```python
from build123d import *

# Parameters (mm, degrees)
SKETCH_1_W             = 26
SKETCH_1_H             = 82
EXTRUDE_1_DEPTH        = 9
CHAMFER_1_SIZE         = 5
CUT_EXTRUDE_1_DEPTH    = 87.492774265
SKETCH_3_OUTSIDE_W     = 45.298
SKETCH_3_OUTSIDE_H     = 101.298
SKETCH_3_OUTSIDE_W_2   = 20
SKETCH_3_OUTSIDE_H_2   = 55
CUT_EXTRUDE_2_DEPTH    = 3
SKETCH_4_W             = 12.420254628
SKETCH_4_H             = 10
CUT_EXTRUDE_3_DEPTH    = 87.492774265
PATTERN_LINEAR_1_COUNT = 4
PATTERN_LINEAR_1_PITCH = 12.5
CUT_EXTRUDE_4_DEPTH    = 87.492774265
SKETCH_6_W             = 12
SKETCH_6_H             = 2
CUT_EXTRUDE_5_DEPTH    = 87.492774265
SKETCH_7_W             = 15
SKETCH_7_H             = 18
CUT_EXTRUDE_6_DEPTH    = 4
CUT_EXTRUDE_7_DEPTH    = 87.492774265
CHAMFER_2_SIZE         = 1
CHAMFER_2_SIZE2        = 2
CHAMFER_3_SIZE2        = 1
CHAMFER_3_SIZE         = 4
CHAMFER_4_SIZE2        = 4
CHAMFER_4_SIZE         = 1
CHAMFER_5_SIZE         = 4.17
CHAMFER_5_SIZE_2       = 4
RIB_1_DEPTH            = 1.5
SKETCH_10_R            = 3.5
CUT_EXTRUDE_8_DEPTH    = 1.5
EXTRUDE_2_DEPTH        = 2
FILLET_1_R             = 4
FILLET_2_R             = 4.5
SKETCH_12_R            = 1
CUT_EXTRUDE_9_DEPTH    = 2
FILLET_1_OF_MIRROR_2_R = 4
FILLET_2_OF_MIRROR_2_R = 4.5
FILLET_3_R             = 1
SKETCH_13_R            = 1.5
CUT_EXTRUDE_11_DEPTH   = 2


# Read off the part's stored shape, not the designer's step: 筋1
# Some blends are built 0.0001 mm under size
with BuildPart() as part:
    # 草图1 → 凸台-拉伸1 (new body)
    with BuildSketch(Plane(origin=(0, 0, 0), x_dir=(0, 0, -1), z_dir=(1, 0, 0))):
        with Locations((13, -41)):
            Rectangle(SKETCH_1_W, SKETCH_1_H)
    extrude(amount=EXTRUDE_1_DEPTH)

    # 倒角1
    chamfer_1_edges = [part.edges().sort_by_distance(p)[0] for p in [
        (9, -41, -26),
        (9, -41, 0),
    ]]
    chamfer(chamfer_1_edges, length=CHAMFER_1_SIZE)

    # 草图2 → 切除-拉伸1 (cut, through all)
    with BuildSketch(Plane.XY):
        Polygon((9, 0), (0, -12.853332061), (0, 0), align=None)
        Polygon((9, -4), (6, -8.28444402), (6, -54.71555598), (9, -59), align=None)
    extrude(amount=-CUT_EXTRUDE_1_DEPTH, mode=Mode.SUBTRACT)

    # 草图3 outside → 切除-拉伸2 (cut)
    with BuildSketch(Plane.ZY):
        with Locations((-13, -41)):
            Rectangle(SKETCH_3_OUTSIDE_W, SKETCH_3_OUTSIDE_H)
        with Locations((-13, -31)):
            Rectangle(SKETCH_3_OUTSIDE_W_2, SKETCH_3_OUTSIDE_H_2, mode=Mode.SUBTRACT)
    extrude(amount=-CUT_EXTRUDE_2_DEPTH, mode=Mode.SUBTRACT)

    # 草图4 → 切除-拉伸3 (cut, through all)
    with BuildSketch(Plane.ZY):
        with Locations((-13, -12)):
            Rectangle(SKETCH_4_W, SKETCH_4_H)
    cut_extrude_3 = extrude(amount=-CUT_EXTRUDE_3_DEPTH, mode=Mode.SUBTRACT)

    # 阵列(线性)1: 切除-拉伸3 ×4
    with Locations(*[(0, -i * PATTERN_LINEAR_1_PITCH, 0) for i in range(1, PATTERN_LINEAR_1_COUNT)]):
        add(cut_extrude_3, mode=Mode.SUBTRACT)

    # 草图5 → 切除-拉伸4 (cut, through all)
    with BuildSketch(Plane.XY):
        Polygon((9, -77), (9, -82), (4.5, -82), align=None)
    extrude(amount=-CUT_EXTRUDE_4_DEPTH, mode=Mode.SUBTRACT)

    # 草图6 → 切除-拉伸5 (cut, through all)
    with BuildSketch(Plane(origin=(9, 0, 0), x_dir=(0, 0, -1), z_dir=(1, 0, 0))):
        with Locations((13, -81)):
            Rectangle(SKETCH_6_W, SKETCH_6_H)
    extrude(amount=-CUT_EXTRUDE_5_DEPTH, mode=Mode.SUBTRACT)

    # 草图7 → 切除-拉伸6 (cut)
    with BuildSketch(Plane.ZY.offset(-3)):
        with Locations((-13, -67.5)):
            Rectangle(SKETCH_7_W, SKETCH_7_H)
    extrude(amount=-CUT_EXTRUDE_6_DEPTH, mode=Mode.SUBTRACT)

    # 草图8 → 切除-拉伸7 (cut, through all)
    with BuildSketch(Plane.XY):
        Polygon((4.5, -82), (3, -80.677124344), (3, -82), align=None)
    extrude(amount=-CUT_EXTRUDE_7_DEPTH, mode=Mode.SUBTRACT)

    # 倒角2
    chamfer_2_edges = [part.edges().sort_by_distance(p)[0] for p in [
        (7, -58.5, -13),
    ]]
    chamfer_2_side = [part.faces().sort_by_distance(p)[0] for p in [
        (3.25, -58.5, -13),
    ]]
    chamfer(chamfer_2_edges, length=CHAMFER_2_SIZE, length2=CHAMFER_2_SIZE2, reference=chamfer_2_side[0])

    # 倒角3
    chamfer_3_edges = [part.edges().sort_by_distance(p)[0] for p in [
        (3, -67.5, -5.5),
    ]]
    chamfer_3_side = [part.faces().sort_by_distance(p)[0] for p in [
        (3.02, -67.5, -5.5),
    ]]
    chamfer(chamfer_3_edges, length=CHAMFER_3_SIZE - 0.0001, length2=CHAMFER_3_SIZE2 - 0.0001, reference=chamfer_3_side[0])  # a hair under: the kernel refuses the full size

    # 倒角4
    chamfer_4_edges = [part.edges().sort_by_distance(p)[0] for p in [
        (3, -67.5, -20.5),
    ]]
    chamfer_4_side = [part.faces().sort_by_distance(p)[0] for p in [
        (3, -67.5, -20.52),
    ]]
    chamfer(chamfer_4_edges, length=CHAMFER_4_SIZE - 0.0001, length2=CHAMFER_4_SIZE2 - 0.0001, reference=chamfer_4_side[0])  # a hair under: the kernel refuses the full size

    # 倒角5
    # the kernel refuses this chamfer: 4.17, 4 mm, written as the material it takes off along each edge
    with BuildSketch(Plane(origin=(3, -76.5, 6.229717564), x_dir=(-0.026903120245147794, -0.9996380455550276, 0), z_dir=(0, 0, -1))) as chamfer_5_piece_1_section:
        Polygon((CHAMFER_5_SIZE * 0.999638045555, -CHAMFER_5_SIZE * 0.0269031202451), (-CHAMFER_5_SIZE_2 * 0.0269031202451, -CHAMFER_5_SIZE_2 * 0.999638045555), (0, 0), align=None)
    chamfer_5_piece_1 = extrude(amount=38.459435128, mode=Mode.PRIVATE)
    chamfer_5_piece_1 = split(chamfer_5_piece_1, bisect_by=Plane(origin=(3.319672902, -80.226492904, -4.580012231), z_dir=(-0.24251850433325217, 0, -0.9701467801605912)), keep=Keep.TOP, mode=Mode.PRIVATE)
    chamfer_5_piece_1 = split(chamfer_5_piece_1, bisect_by=Plane(origin=(7.071862718, -80.226492904, -20.48201067), z_dir=(-0.24251850433325217, 0, 0.9701467801605912)), keep=Keep.TOP, mode=Mode.PRIVATE)
    add(chamfer_5_piece_1, mode=Mode.SUBTRACT)

    # 筋1 outline → 筋1 (add)
    with BuildSketch(Plane.XY.offset(-10.5)):
        Polygon((0, -74), (0, -80), (3.642685851, -80), (7, -76.5), (7, -73.5), align=None)
    rib_1 = extrude(amount=RIB_1_DEPTH)

    # 草图10 → 切除-拉伸8 (cut)
    with BuildSketch(Plane(origin=(0, 0, -10.5), x_dir=(-1, 0, 0), z_dir=(0, 0, -1))):
        with Locations((3, -77)):
            Circle(SKETCH_10_R)
    cut_extrude_8 = extrude(amount=-CUT_EXTRUDE_8_DEPTH, mode=Mode.SUBTRACT)

    # 镜向1: 筋1, 切除-拉伸8 across plane
    add(rib_1.mirror(Plane.XY.offset(-13)))
    add(cut_extrude_8.mirror(Plane.XY.offset(-13)), mode=Mode.SUBTRACT)

    # 草图11 → 凸台-拉伸2 (add)
    with BuildSketch(Plane(origin=(0, 0, -26), x_dir=(-1, 0, 0), z_dir=(0, 0, -1))):
        with BuildLine():
            Line((-3, -80.677124344), (-3, -73.177124344))
            Line((-3, -73.177124344), (7, -73.177124344))
            Line((7, -73.177124344), (7, -85.177124344))
            Line((7, -85.177124344), (4.616572218, -85.177124344))
            Line((4.616572218, -85.177124344), (4.616572218, -83.177124344))
            ThreePointArc((4.616572218, -83.177124344), (1.349260187, -80.278977091), (-3, -80.677124344))
        make_face()
    extrude_2 = extrude(amount=-EXTRUDE_2_DEPTH)

    # 圆角1
    fillet_1_edges = [part.edges().sort_by_distance(p)[0] for p in [
        (-7, -73.177124344, -25),
    ]]
    fillet(fillet_1_edges, radius=FILLET_1_R)

    # 圆角2
    # the kernel refuses this fillet: 4.5 mm, written as the material it takes off along each edge
    with BuildSketch(Plane(origin=(-7, -85.177124344, -35.927903243), x_dir=(0, 1, 0), z_dir=(0, 0, 1))) as fillet_2_piece_1:
        with BuildLine():
            CenterArc((3.971161297, -4.5), FILLET_2_R, 90, 61.943021953)
            Line((0, -2.383427782), (-0.079423226, -2.341096338))
            ThreePointArc((-0.079423226, -2.341096338), (-0.09, -1.191713891), (-0.09, 0))
            Line((-0.09, 0), (0, 0.09))
            Line((0, 0.09), (3.971161297, 0.09))
            Line((3.971161297, 0.09), (3.971161297, 0))
        make_face()
    extrude(amount=21.855806485, mode=Mode.SUBTRACT)

    # 草图12 → 切除-拉伸9 (cut)
    with BuildSketch(Plane(origin=(0, 0, -26), x_dir=(-1, 0, 0), z_dir=(0, 0, -1))):
        with Locations(Location((2.5, -77.177124344, 0), (0, 0, 90))):
            Circle(SKETCH_12_R)
    cut_extrude_9 = extrude(amount=-CUT_EXTRUDE_9_DEPTH, mode=Mode.SUBTRACT)

    # 镜向2: 凸台-拉伸2, 切除-拉伸9 across plane
    add(extrude_2.mirror(Plane.XY.offset(-13)))
    add(cut_extrude_9.mirror(Plane.XY.offset(-13)), mode=Mode.SUBTRACT)

    # 圆角1 of 镜向2
    fillet_1_of_mirror_2_edges = [part.edges().sort_by_distance(p)[0] for p in [
        (-7, -73.177124344, -1),
    ]]
    fillet(fillet_1_of_mirror_2_edges, radius=FILLET_1_OF_MIRROR_2_R)

    # 圆角2 of 镜向2
    # the kernel refuses this fillet: 4.5 mm, written as the material it takes off along each edge
    with BuildSketch(Plane(origin=(-7, -85.177124344, 9.927903243), x_dir=(0, 1, 0), z_dir=(0, 0, -1))) as fillet_2_of_mirror_2_piece_1:
        with BuildLine():
            CenterArc((3.971161297, 4.5), FILLET_2_OF_MIRROR_2_R, 208.056978047, 61.943021953)
            Line((0, 2.383427782), (-0.079423226, 2.341096338))
            ThreePointArc((-0.079423226, 2.341096338), (-0.09, 1.191713891), (-0.09, 0))
            Line((-0.09, 0), (0, -0.09))
            Line((0, -0.09), (3.971161297, -0.09))
            Line((3.971161297, -0.09), (3.971161297, 0))
        make_face()
    extrude(amount=21.855806485, mode=Mode.SUBTRACT)

    # 圆角3
    # the kernel refuses this fillet: 1 mm, written as the material it takes off along each edge
    with BuildSketch(Plane(origin=(-4.616572218, -85.177124344, -32.450380338), x_dir=(-0.7105970280063522, 0.7035992209976782, 0), z_dir=(0, 0, 1))) as fillet_3_piece_1:
        with BuildLine():
            CenterArc((2.293468564, -0.958025329), FILLET_3_R, 73.340489996, 134.251279475)
            Line((1.407198442, -1.421194056), (1.38947304, -1.430457431))
            ThreePointArc((1.38947304, -1.430457431), (0.68938728, -0.724669012), (-0.014211941, -0.014071984))
            Line((-0.014211941, -0.014071984), (-0.005733671, 0.019160507))
            ThreePointArc((-0.005733671, 0.019160507), (1.290076068, 0.208886021), (2.585885806, 0.019160507))
            Line((2.585885806, 0.019160507), (2.580152135, 0))
        make_face()
    extrude(amount=14.900760675, mode=Mode.SUBTRACT)
    with BuildSketch(Plane(origin=(-4.616572218, -85.177124344, 6.450380338), x_dir=(0, 1, 0), z_dir=(0, 0, -1))) as fillet_3_piece_2:
        with BuildLine():
            CenterArc((2.294452647, -0.955666071), FILLET_3_R, 107.12471858, 134.251279475)
            Line((1.815393032, -1.833448439), (1.80581184, -1.851004086))
            ThreePointArc((1.80581184, -1.851004086), (0.75926273, -1.063696261), (-0.017649606, -0.009406988))
            Line((-0.017649606, -0.009406988), (0, 0.02))
            ThreePointArc((0, 0.02), (1, 0.02), (1.994110947, 0.019113321))
            Line((1.994110947, 0.019113321), (2, 0))
        make_face()
    extrude(amount=14.900760675, mode=Mode.SUBTRACT)

    # 草图13 → 切除-拉伸11 (cut)
    with BuildSketch(Plane(origin=(0, 0, -26), x_dir=(-1, 0, 0), z_dir=(0, 0, -1))):
        with Locations(Location((2.5, -77.177124344, 0), (0, 0, 90))):
            Circle(SKETCH_13_R)
    extrude(amount=-CUT_EXTRUDE_11_DEPTH, mode=Mode.SUBTRACT)


solid = part.part
```
Build history of the part. All positions in model axes, mm. A direction names the side the tool comes from. Coordinates: 2 decimals unless noted, no trailing zeros. Order: outer loops, then holes, each group sorted by start corner. A loop starts at its lowest first (then second) coordinate and runs counter-clockwise, first axis right, second up. Notation, with made-up numbers: (60.25, -30) -> (105.25, -30) arc R25 ccw to (105.25, 3) -> close; hole circle Ø5 at (3, 8). An arc over 180 degrees is marked (long way). Answer in a Markdown table with one row per item. Add a question column.
Q1. Wall check: line 1 along Z through (x, y) = (3.5, -16); line 2 along Z through (x, y) = (4.5, -25.5); line 3 along X through (y, z) = (-50.5, -5). Give the ranges that are in metal, low to high. Write a range as [from, to].
Q2. Band-saw the part on A-A, the plane y = -33.5. List the corners of the cut face in (x, z).
Q3. Drop flat-ended pins along their axis: pin 1 (3 mm diameter, centred on x = 6, z = -10.5, fed in from -Y); pin 2 (2 mm diameter, centred on x = -0.5, y = -12.5, fed in from -Z); pin 3 (2 mm diameter, centred on x = 0.5, z = -25, fed in from +Y). Give the stop position or say it passes through.
Q4. Which spindle directions (+Z, -Z, +X, -X, +Y, -Y) get a long thin tool onto all of the face, cutting with end or side? Do faces 4 (the face through (-1, -78, -24)), 5 (the face through (3.76, -81.35, -22.45)), 6 (the face through (4.972, -78.614, -19.218)), 7 (the face through (3, -25, -19.21)). Say none if no direction does.
Q5. Mould opens along X. For faces 1 (the face through (5, -51, -1)), 2 (the face through (3.76, -81.35, -3.45)), 3 (the face through (-6.856, -82.334, -0.986)) say: +X half, -X half, draft (parallel to the pull), parting line (faces both ways), or undercut.
Q6. Band-saw the part on B-B, the plane z = -22.25. List the corners of the cut face in (x, y).
Answers follow:
| question | item | result |
|---|---|---|
| 1 | line 1 | [-26, -19.21], [-6.79, 0] |
| 1 | line 2 | [-25.5, -19.21], [-6.79, -0.5] |
| 1 | line 3 | [0, 6] |
| 2 | outline | (0, -23) -> (3, -23) -> (3, -26) -> (4, -26) -> (6, -24) -> (6, -19.21) -> (0, -19.21) -> close; (0, -6.79) -> (6, -6.79) -> (6, -2) -> (4, 0) -> (3, 0) -> (3, -3) -> (0, -3) -> close |
| 3 | pin 1 | y = -80 |
| 3 | pin 2 | z = -23 |
| 3 | pin 3 | y = -73.18 |
| 4 | face 4 | -X, +Y, -Y |
| 4 | face 5 | +Z, -Z, -Y |
| 4 | face 6 | -X |
| 4 | face 7 | +X, -X |
| 5 | face 1 | +X half |
| 5 | face 2 | undercut |
| 5 | face 3 | -X half |
| 6 | outline | (0, -58.5) -> (3, -58.5) -> (3, -80.68) -> (4.5, -82) -> (7.75, -78.39) -> (7.75, -57.21) -> (6, -54.72) -> (6, -8.28) -> (7.75, -5.79) -> (7.75, -1.79) -> (0, -12.85) -> close |
